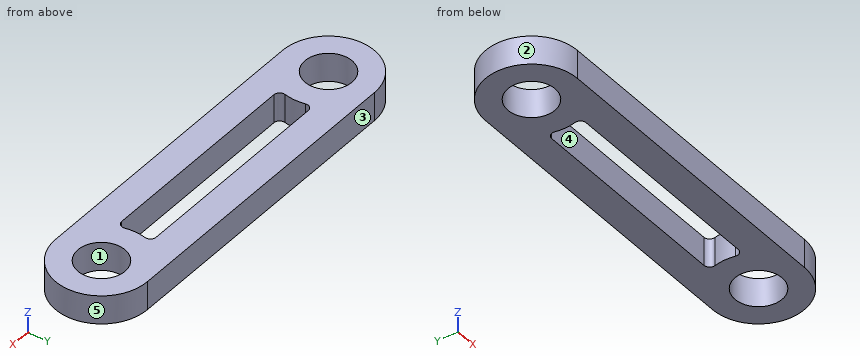
Solid Edge part; units mm, degrees
sketch "Sketch1" plane through (0, 0, 0) normal (0, 0, 1) x (1, 0, 0)
  circle A0 centre (-17.4781, 0) radius 4.1
  line L0 (-17.4781, 8) -> (35.7219, 8)
  line L1 (35.7219, -8) -> (-17.4781, -8)
  arc A1 (-17.4781, -8) -> (-17.4781, 8) centre (-17.4781, 0) cw
  arc A2 (35.7219, 8) -> (35.7219, -8) centre (35.7219, 0) cw
  line L2 (-8.7031, 3) -> (26.9469, 3)
  arc A3 (27.9219, 1.7778) -> (26.9469, 3) centre (26.9469, 2) ccw
  arc A4 (27.9219, -1.7778) -> (27.9219, 1.7778) centre (35.7219, 0) cw
  arc A5 (26.9469, -3) -> (27.9219, -1.7778) centre (26.9469, -2) ccw
  line L3 (26.9469, -3) -> (-8.7031, -3)
  arc A6 (-9.6781, -1.7778) -> (-8.7031, -3) centre (-8.7031, -2) ccw
  arc A7 (-9.6781, 1.7778) -> (-9.6781, -1.7778) centre (-17.4781, 0) cw
  arc A8 (-8.7031, 3) -> (-9.6781, 1.7778) centre (-8.7031, 2) ccw
  circle A9 centre (35.7219, 0) radius 4.1
extrude "Protrusion1" add sketch "Sketch1" along normal blind 5
extrude "Cutout1" [suppressed]
extrude "ExtrudedProtrusion_2" [suppressed]
Input: part model. Units: mm. Frame: model coordinates. Face numbers are marked on the shaded views. A direction names the side the tool comes from. Coordinates: 2 decimals unless noted, no trailing zeros. Order: outer loops, then holes, each group sorted by start corner. A loop starts at its lowest first (then second) coordinate and runs counter-clockwise, first axis right, second up. Notation, with made-up numbers: (62, 23.25) - (66, 23.25) arc R23 cw to (66, 60.25) - close; hole circle Ø5 at (-7.75, 8). An arc over 180 degrees is marked (long way). Return JSON: item names as keys, results as strings.
Q1. Cut plane A-A (y = 0). Return loops of the section in (x, z).
The answers:
{"outline": "(-25.48, 0) - (-21.58, 0) - (-21.58, 5) - (-25.48, 5) - close; (-13.38, 0) - (-9.48, 0) - (-9.48, 5) - (-13.38, 5) - close; (27.72, 0) - (31.62, 0) - (31.62, 5) - (27.72, 5) - close; (39.82, 0) - (43.72, 0) - (43.72, 5) - (39.82, 5) - close"}
Q2. First-contact query: pin 1 (1 mm diameter, centred on y = -4.5, z = 1, fed in from -X); pin 2 (1 mm diameter, centred on y = -4.5, z = 3, fed in from +X). Flat tips, straight axial feed; report the tip coordinate or a pass-through.
The answers:
{"pin 1": "stops at x = -24.41", "pin 2": "stops at x = 42.65"}
Q3. Cut plane B-B (x = 35). Return loops of the section in (y, z), then the cut area to 3 significant figures.
The answers:
{"outline": "(-8, 0) - (-4.04, 0) - (-4.04, 5) - (-8, 5) - close; (4.04, 0) - (8, 0) - (8, 5) - (4.04, 5) - close", "area": "39.6 mm2"}
Q4. Access query for the marked faces 4 and 5. Directions: +Z, -Z, +X, -X, +Y, -Y. A direction counts if a zero-diameter tool reaches every point of the face in a straight line with its end or side. Return the directions, or none.
The answers:
{"face 4": "+Z, -Z", "face 5": "+Z, -Z, +X"}
Q5. Draft query along X for the marked faces 1, 2 and 3. Return one class per face: +X half, -X half, draft (parallel to the pull), parting line (faces both ways), or undercut.
The answers:
{"face 1": "undercut", "face 2": "-X half", "face 3": "draft"}
Q6. Cut plane D-D (y = 7). Return loops of the section in (x, z).
The answers:
{"outline": "(-21.35, 0) - (39.59, 0) - (39.59, 5) - (-21.35, 5) - close"}
Q7. Cut plane C-C (z = 3.3). Return loops of the section in (x, y), then the cut area to 3 significant figures.
The answers:
{"outline": "(-17.48, -8) - (35.72, -8) arc R8 ccw to (35.72, 8) - (-17.48, 8) arc R8 ccw to start; hole circle Ø8.2 at (-17.48, 0); hole (-9.68, -1.78) arc R1 ccw to (-8.7, -3) - (26.95, -3) arc R1 ccw to (27.92, -1.78) arc R8 cw to (27.92, 1.78) arc R1 ccw to (26.95, 3) - (-8.7, 3) arc R1 ccw to (-9.68, 1.78) arc R8 cw to start; hole circle Ø8.2 at (35.72, 0)", "area": "723 mm2"}
Q8. Ray query, probe 1 along Y at (x, z) = (9.5, 3.8); probe 2 along X at (y, z) = (-0.5, 1.7); probe 3 along X at (y, z) = (-3.75, 3.1). Return the intervals inside material, ascending.
The answers:
{"probe 1": "y = -8 to -3, 3 to 8", "probe 2": "x = -25.46 to -21.55, -13.41 to -9.49, 27.74 to 31.65, 39.79 to 43.71", "probe 3": "x = -24.54 to -19.14, -15.82 to 34.06, 37.38 to 42.79"}
